Verification items for the finished model (mm, model axes). Face numbers are marked on the shaded views. A direction names the side the tool comes from. Coordinates: 2 decimals unless noted, no trailing zeros. Order: outer loops, then holes, each group sorted by start corner. A loop starts at its lowest first (then second) coordinate and runs counter-clockwise, first axis right, second up. Notation, with made-up numbers: M 87.25,6 L 94.25,6 A33 ccw 94.25,36 Z; hole C -24,84 d5. An arc over 180 degrees is marked long. Use one line per item in the form item = value. Start each with the question number.
Autodesk Fusion 360 part; units mm, degrees
sketch "Sketch1" plane through (0, 0, 0) normal (0, 0, 1) x (1, 0, 0)
  circle A0 centre (0, 0) radius 2
  circle A1 centre (0, 0) radius 3.5
  circle A2 centre (-10, -24) radius 2
  circle A3 centre (-10, -24) radius 3.25
  line L0 (-10, -24) -> (-10, -20.75) construction
  line L1 (-10, -20.75) -> (-10, -18.9342)
  line L2 (0, 0) -> (0, -3.5) construction
  line L3 (-9.4696, -17.231) -> (0, -3.5)
  line L4 (-10, -24) -> (-10, -27.25) construction
  line L5 (-10, -27.25) -> (-10, -33)
  circle A4 centre (-12, -33) radius 2
  line L6 (-14, -33) -> (-14, -19.8683)
  line L7 (-12.9393, -16.462) -> (-2.9185, -1.9319)
  arc A5 (-12.9393, -16.462) -> (-14, -19.8683) centre (-8, -19.8683) ccw
  arc A6 (-9.4696, -17.231) -> (-10, -18.9342) centre (-7, -18.9342) ccw
  point P0 (-10, -18)
  point P1 (-14, -18)
  dimension "d1" = 4
  dimension "d2" = 7
  dimension "d3" = 4
  dimension "d4" = 24
  dimension "d5" = 10
  dimension "d6" = 6.5
  dimension "d7" = 2.75
  dimension "d8" = 4
  dimension "d9" = 5.75
  dimension "d11" = 15
  dimension "d12" = 4
  dimension "d13" = 6
  dimension "d14" = 3
extrude "Extrude1" add sketch "Sketch1" along normal blind 4 contours A1 | A1 A3 L1 L3 L5 A4 L6 L7 A5 A6 | A4
extrude "Extrude2" add sketch "Sketch1" along normal blind 2 contours A3
extrude "Extrude3" add sketch "Sketch1" along normal blind 4 contours A2
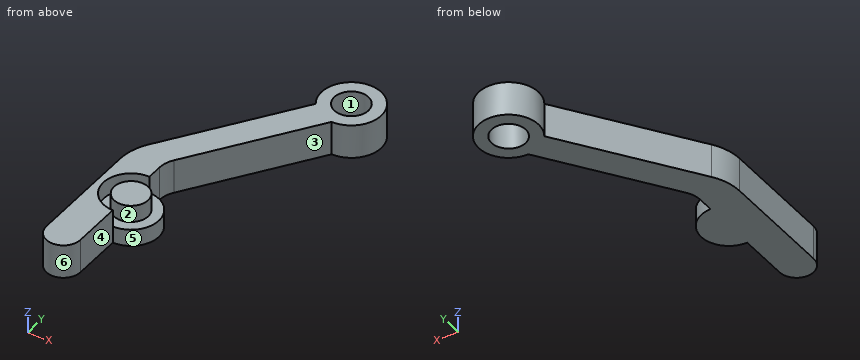
1. Cross-section at A-A on z = 2.6. Enter the section's corners in (x, y), and give its area (3 significant figures).
2. Cross-section at C-C on y = -24. Enter the section's corners in (x, z).
3. Depth check by flat-ended pin: P1, Ø2, axis at x = -0.5, z = 3, coming from the -Y side (3 decimals); P2, Ø1.2, axis at y = -30.5, z = 1.5, coming from the +X side; P3, Ø2, axis at x = -1.5, z = 0.5, coming from the +Y side. Enter the tip coordinate at first touch or a pass-through.
4. Cross-section at B-B on y = 0. Enter the section's corners in (x, z), and give its area (3 significant figures).
5. Release check for a two-part mould opening along Y. For the marked faces 4, 5 and 6 record: pulls with the +Y half, pulls with the -Y half, needs draft (parallel to the pull), parting line crosses it, or undercut.
6. Tool access check on the marked faces 1, 2 and 3. Record the directions out of +Z, -Z, +X, -X, +Y, -Y that give a thin tool (end or side, any length) a straight path to the whole face; none if there is none.
7. Material ranges on line 1 along X through (y, z) = (-29.5, 2); line 2 along Y through (x, z) = (-12.5, 3.8); line 3 along Z through (x, y) = (-12.25, -24), recorded low to high.
8. Cross-section at D-D on y = -4. Enter the section's corners in (x, z), and give its area (3 significant figures).
Final values:
q1.outline = M -14,-33 A2 ccw -10,-33 L -10,-27.25 A3.25 cw -10,-20.75 L -10,-18.93 A3 cw -9.47,-17.23 L 0,-3.5 A3.5 ccw long -2.92,-1.93 L -12.94,-16.46 A6 ccw -14,-19.87 Z; C -10,-24 d4; hole C 0,0 d4
q1.area = 148 mm2
q2.outline = M -14,0 L -6.75,0 L -6.75,2 L -8,2 L -8,4 L -12,4 L -12,2 L -13.25,2 L -13.25,4 L -14,4 Z
q3.P1 = -5.675
q3.P2 = -10
q3.P3 = 3.46
q4.outline = M -3.5,0 L -2,0 L -2,4 L -3.5,4 Z; M 2,0 L 3.5,0 L 3.5,4 L 2,4 Z
q4.area = 12.0 mm2
q5.face_4 = needs draft
q5.face_5 = undercut
q5.face_6 = pulls with the -Y half
q6.face_1 = +Z, -Z
q6.face_2 = +Z
q6.face_3 = +Z, -Z, +X
q7.line_1 = -14 to -10
q7.line_2 = -34.94 to -26.08, -21.92 to -15.83
q7.line_3 = 0 to 2
q8.outline = M -4.34,0 L -0.34,0 L -0.34,4 L -4.34,4 Z
q8.area = 16.0 mm2
